Geometry check sheet. Reference: the model listing, model coordinates, mm. Face numbers are marked on the shaded views. Coordinates: 2 decimals unless noted, no trailing zeros. Write each loop counter-clockwise with the first axis right and the second up, starting at its lowest first coordinate (ties: lowest second). Pieces come first, ordered by that corner, then holes.
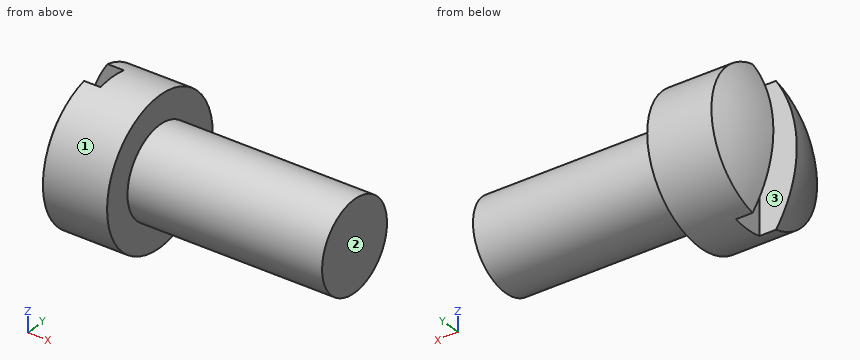
from build123d import *

# Parameters (mm, degrees)
SKETCH2_W  = 3.556
SKETCH2_H  = 0.7874
SLOT_DEPTH = 0.9398


with BuildPart() as part:
    # BodySke → Base-Revolve (revolve)
    with BuildSketch(Plane.XY, mode=Mode.PRIVATE) as base_revolve_sk:
        with BuildLine():
            Line((2.1082, 1.0922), (2.1082, 1.778))
            Line((2.1082, 1.778), (0.5334, 1.778))
            ThreePointArc((0.5334, 1.778), (0.136222505, 0.928143249), (0, 0))
            Line((0, 0), (6.8834, 0))
            Line((6.8834, 0), (6.8834, 1.0922))
            Line((6.8834, 1.0922), (2.1082, 1.0922))
        make_face()
    revolve(base_revolve_sk.sketch.rotate(Axis((-9.603521982, 0, 0), (1, 0, 0)), 90), axis=Axis((-9.603521982, 0, 0), (1, 0, 0)))  # turned: the seam where the file's is

    # Sketch2 → Slot (cut)
    with BuildSketch(Plane(origin=(0, 0, 0), x_dir=(0, 0, -1), z_dir=(1, 0, 0))):
        Rectangle(SKETCH2_W, SKETCH2_H)
    extrude(amount=SLOT_DEPTH, mode=Mode.SUBTRACT)


solid = part.part
1. Sectioned sample at A-A, the plane y = 0. Record the boundary of the cut face in (x, z), and give its area (3 significant figures).
Computed values:
outline: (0.94, -1.78) - (2.11, -1.78) - (2.11, -1.09) - (6.88, -1.09) - (6.88, 1.09) - (2.11, 1.09) - (2.11, 1.78) - (0.94, 1.78) - close
area: 14.6 mm2
2. Sectioned sample at B-B, the plane z = 0. Record the boundary of the cut face in (x, y).
Computed values:
outline: (0.02, -0.39) arc R3.23 ccw to (0.53, -1.78) - (2.11, -1.78) - (2.11, -1.09) - (6.88, -1.09) - (6.88, 1.09) - (2.11, 1.09) - (2.11, 1.78) - (0.53, 1.78) arc R3.23 ccw to (0.02, 0.39) - (0.94, 0.39) - (0.94, -0.39) - close
3. Sectioned sample at D-D, the plane z = 1.4. Record the boundary of the cut face in (x, y), and give its area (3 significant figures).
Computed values:
outline: (0.35, -0.39) arc R2.91 ccw to (0.53, -1.1) - (2.11, -1.1) - (2.11, 1.1) - (0.53, 1.1) arc R2.91 ccw to (0.35, 0.39) - (0.94, 0.39) - (0.94, -0.39) - close
area: 3.29 mm2
4. Sectioned sample at C-C, the plane x = 2. Record the boundary of the cut face in (y, z), and give its area (3 significant figures).
Computed values:
outline: circle Ø3.56 at (0, 0)
area: 9.93 mm2
5. Thickness scan on line 1 along X through (y, z) = (0.1, -1.2); line 2 along Y through (x, z) = (0.75, -1.5); line 3 along X through (y, z) = (0, -1). Record the ranges inside material, lowest first.
Computed values:
line 1: x = 0.94 to 2.11
line 2: y = -0.95 to -0.39, 0.39 to 0.95
line 3: x = 0.94 to 6.88
6. Draft check along Y on the marked faces 1, 2 and 3. Enter one of: released by +Y, released by -Y, zero draft, split by the parting line, or undercut.
Computed values:
face 1: split by the parting line
face 2: zero draft
face 3: undercut
7. Gauge pin test, flat ends, axial feed: pin 1 Ø0.7 at (x, z) = (0.5, 1) entering from -Y; pin 2 Ø1 at (y, z) = (0.5, -1) entering from -X. Record the tip position at first contact, or that the pin passes through.
Computed values:
pin 1: stops at y = -1.65
pin 2: stops at x = 0.07
